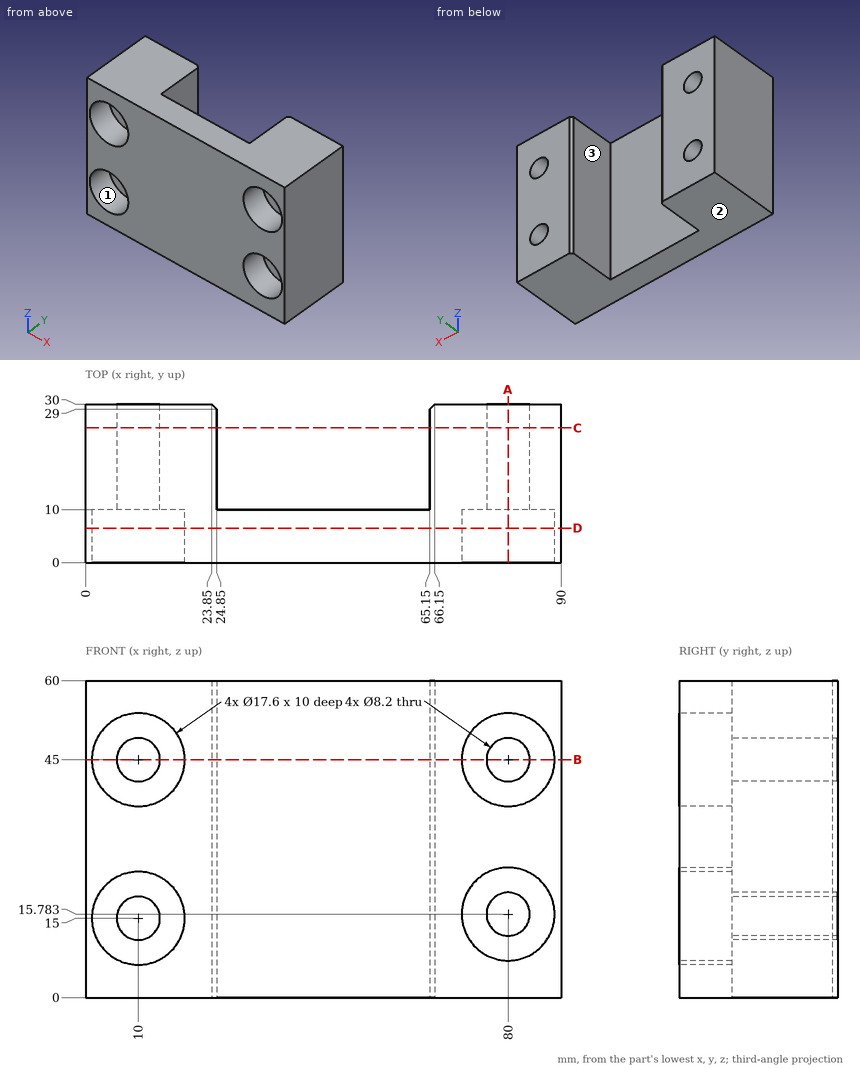
Check sheet for the drawn part. Datum: minimum x, y, z corner. Units: mm. A direction names the side the tool comes from. Round coordinates to 2 decimals unless told otherwise and drop trailing zeros. Order: outer loops, then holes, each group sorted by start corner. A loop starts at its lowest first (then second) coordinate and runs counter-clockwise, first axis right, second up.
(1) Go/stop test with a flat-tipped pin: P1, Ø9.5, axis at x = 10, z = 15, coming from the -Y side. Record where the tip stops, or that it passes through.
(2) Cross-section at B-B, the plane z = 45. Enter the section's corners in (x, y).
(3) Cross-section at D-D, the plane y = 6.5. Enter the section's corners in (x, z), and give its area (3 significant figures).
(4) Scan lines: probe 1 along Z at (x, y) = (10, 17); probe 2 along Z at (x, y) = (80, 17); probe 3 along X at (y, z) = (11.5, 38). Record each from-to range of solid material in increasing order.
(5) Access from +Z, -Z, +X, -X, +Y, -Y to the whole of each face (thin tool, end or side, straight path). Record for the marked faces 1, 2 and 3.
(6) Cross-section at C-C, the plane y = 25.5. Enter the section's corners in (x, z).
(7) Cross-section at A-A, the plane x = 80. Enter the section's corners in (y, z), and give its area (3 significant figures).
Check sheet entries:
1. P1: stops at y = 10
2. outline: (0, 0) - (1.2, 0) - (1.2, 10) - (5.9, 10) - (5.9, 30) - (0, 30) - close; (14.1, 10) - (18.8, 10) - (18.8, 0) - (71.2, 0) - (71.2, 10) - (75.9, 10) - (75.9, 30) - (66.15, 30) - (65.15, 29) - (65.15, 10) - (24.85, 10) - (24.85, 29) - (23.85, 30) - (14.1, 30) - close; (84.1, 10) - (88.8, 10) - (88.8, 0) - (90, 0) - (90, 30) - (84.1, 30) - close
3. outline: (0, 0) - (90, 0) - (90, 60) - (0, 60) - close; hole circle Ø17.6 at (10, 15); hole circle Ø17.6 at (10, 45); hole circle Ø17.6 at (80, 15.78); hole circle Ø17.6 at (80, 45)
3. area: 4,430 mm2
4. probe 1: z = 0 to 10.9, 19.1 to 40.9, 49.1 to 60
4. probe 2: z = 0 to 11.68, 19.88 to 40.9, 49.1 to 60
4. probe 3: x = 0 to 24.85, 65.15 to 90
5. face 1: -Y
5. face 2: -Z, +X, -X, +Y, -Y
5. face 3: +Z, -Z, +Y
6. outline: (0, 0) - (24.85, 0) - (24.85, 60) - (0, 60) - close; (65.15, 0) - (90, 0) - (90, 60) - (65.15, 60) - close; hole circle Ø8.2 at (10, 15); hole circle Ø8.2 at (10, 45); hole circle Ø8.2 at (80, 15.78); hole circle Ø8.2 at (80, 45)
7. outline: (0, 0) - (30, 0) - (30, 11.68) - (10, 11.68) - (10, 6.98) - (0, 6.98) - close; (0, 24.58) - (10, 24.58) - (10, 19.88) - (30, 19.88) - (30, 40.9) - (10, 40.9) - (10, 36.2) - (0, 36.2) - close; (0, 53.8) - (10, 53.8) - (10, 49.1) - (30, 49.1) - (30, 60) - (0, 60) - close
7. area: 1,120 mm2
